Geometry: final body of the model. Coordinates: model frame, mm. Face numbers are marked on the shaded views. A direction names the side the tool comes from. Coordinates: 2 decimals unless noted, no trailing zeros. Order: outer loops, then holes, each group sorted by start corner. A loop starts at its lowest first (then second) coordinate and runs counter-clockwise, first axis right, second up. Notation, with made-up numbers: (58, -32.5) - (71, -32.5) arc R36 cw to (71, 6.5) - close; hole circle Ø11 at (48.25, 27.5). An arc over 180 degrees is marked (long way). Use one line per item in the form item = value. Start each with the question number.
```python
from build123d import *

# Parameters (mm, degrees)
SKETCH1_W                 = 50.8
SKETCH1_H                 = 50.8
SKETCH1_W_2               = 38.1
SKETCH1_H_2               = 38.1
BOSS_EXTRUDE1_DEPTH       = 178
SKETCH2_W                 = 44.8
SKETCH2_H                 = 44.8
SKETCH2_W_2               = 38.1
SKETCH2_H_2               = 38.1
CUT_EXTRUDE1_DEPTH        = 20
SKETCH3_W                 = 46.8
SKETCH3_H                 = 123.47500012
CUT_EXTRUDE2_DEPTH        = 47.625
CUT_EXTRUDE5_DEPTH        = 1
SKETCH7_W                 = 46.8
SKETCH7_H                 = 3.675
CUT_EXTRUDE6_DEPTH        = 1
FILLET1_R                 = 1.5875
CUT_EXTRUDE7_REACH        = 193.951
F_0_80_TAPPED_HOLE1_D     = 1.19126
F_0_80_TAPPED_HOLE1_DEPTH = 2.9997
F_0_80_TAPPED_HOLE1_TIP   = 0.357890611
SKETCH19_W                = 50.8
SKETCH19_H                = 1.5875
CUT_EXTRUDE12_DEPTH       = 4
CIRPATTERN1_COUNT         = 4
CUT_EXTRUDE13_DEPTH       = 191.931610793
LPATTERN1_COUNT           = 2
LPATTERN1_PITCH           = 8.41
LPATTERN1_COPY_1_SKETCH_W = 50.8
LPATTERN1_COPY_1_SKETCH_H = 1.5875
LPATTERN1_COPY_1_DEPTH    = 4
LPATTERN1_COPY_2_SKETCH_W = 50.8
LPATTERN1_COPY_2_SKETCH_H = 1.5875
LPATTERN1_COPY_2_DEPTH    = 4
LPATTERN1_COPY_3_SKETCH_W = 50.8
LPATTERN1_COPY_3_SKETCH_H = 1.5875
LPATTERN1_COPY_3_DEPTH    = 4


with BuildPart() as part:
    # Sketch1 → Boss-Extrude1 (new body)
    with BuildSketch(Plane(origin=(0, 0, 0), x_dir=(1, 0, 0), z_dir=(0, 1, 0))):
        with Locations((25.4, 25.4)):
            Rectangle(SKETCH1_W, SKETCH1_H)
        with Locations((25.4, 25.4)):
            Rectangle(SKETCH1_W_2, SKETCH1_H_2, mode=Mode.SUBTRACT)
    extrude(amount=BOSS_EXTRUDE1_DEPTH)

    # Sketch2 → Cut-Extrude1 (cut)
    with BuildSketch(Plane.XZ):
        with Locations((25.4, -25.4)):
            Rectangle(SKETCH2_W, SKETCH2_H)
        with Locations((25.4, -25.4)):
            Rectangle(SKETCH2_W_2, SKETCH2_H_2, mode=Mode.SUBTRACT)
    extrude(amount=-CUT_EXTRUDE1_DEPTH, mode=Mode.SUBTRACT)

    # Sketch3 → Cut-Extrude2 (cut)
    with BuildSketch(Plane.XY):
        with Locations((25.4, 109.41249994)):
            Rectangle(SKETCH3_W, SKETCH3_H)
    extrude(amount=-CUT_EXTRUDE2_DEPTH, mode=Mode.SUBTRACT)

    # Sketch6 → Cut-Extrude5 (cut)
    with BuildSketch(Plane.ZY):
        with BuildLine():
            Line((-32.4, 171.5), (-18.4, 171.5))
            ThreePointArc((-18.4, 171.5), (-17.4, 170.5), (-18.4, 169.5))
            Line((-18.4, 169.5), (-32.4, 169.5))
            ThreePointArc((-32.4, 169.5), (-33.4, 170.5), (-32.4, 171.5))
        make_face()
        with BuildLine():
            Line((-32.4, 168), (-18.4, 168))
            ThreePointArc((-18.4, 168), (-17.4, 167), (-18.4, 166))
            Line((-18.4, 166), (-32.4, 166))
            ThreePointArc((-32.4, 166), (-33.4, 167), (-32.4, 168))
        make_face()
        with BuildLine():
            Line((-32.4, 164.5), (-18.4, 164.5))
            ThreePointArc((-18.4, 164.5), (-17.4, 163.5), (-18.4, 162.5))
            Line((-18.4, 162.5), (-32.4, 162.5))
            ThreePointArc((-32.4, 162.5), (-33.4, 163.5), (-32.4, 164.5))
        make_face()
    cut_extrude5 = extrude(amount=-CUT_EXTRUDE5_DEPTH, mode=Mode.SUBTRACT)

    # Mirror2: Cut-Extrude5 across plane
    add(cut_extrude5.mirror(Plane.ZY.offset(-25.4)), mode=Mode.SUBTRACT)

    # Sketch7 → Cut-Extrude6 (cut)
    with BuildSketch(Plane.XY):
        with Locations((25.4, 172.9875)):
            Rectangle(SKETCH7_W, SKETCH7_H)
        with Locations((25.4, 45.83749988)):
            Rectangle(SKETCH7_W, SKETCH7_H)
    extrude(amount=-CUT_EXTRUDE6_DEPTH, mode=Mode.SUBTRACT)

    # Fillet1
    fillet1_edges = [part.edges().sort_by_distance(p)[0] for p in [
        (2, 174.825, -0.5),
        (48.8, 174.825, -0.5),
        (2, 43.99999988, -0.5),
        (48.8, 43.99999988, -0.5),
        (47.8, 10, -3),
        (47.8, 10, -47.8),
        (3, 10, -47.8),
        (3, 10, -3),
        (2, 47.67499988, -24.3125),
        (2, 171.15, -24.3125),
        (48.8, 171.15, -24.3125),
        (48.8, 47.67499988, -24.3125),
    ]]
    fillet(fillet1_edges, radius=FILLET1_R)

    # Sketch8 → Cut-Extrude7 (cut, up to next)
    with BuildSketch(Plane(origin=(0, 178, 0), x_dir=(1, 0, 0), z_dir=(0, 1, 0)), mode=Mode.PRIVATE) as cut_extrude7_sk1:
        with BuildLine():
            Line((6.9375, 45.45), (43.8625, 45.45))
            ThreePointArc((43.8625, 45.45), (44.985032015, 44.985032015), (45.45, 43.8625))
            Line((45.45, 43.8625), (45.45, 6.9375))
            ThreePointArc((45.45, 6.9375), (44.985032015, 5.814967985), (43.8625, 5.35))
            Line((43.8625, 5.35), (6.9375, 5.35))
            ThreePointArc((6.9375, 5.35), (5.814967985, 5.814967985), (5.35, 6.9375))
            Line((5.35, 6.9375), (5.35, 43.8625))
            ThreePointArc((5.35, 43.8625), (5.814967985, 44.985032015), (6.9375, 45.45))
        make_face()
    cut_extrude7_tool1 = extrude(cut_extrude7_sk1.sketch, amount=-CUT_EXTRUDE7_REACH, mode=Mode.PRIVATE) & part.part
    add(cut_extrude7_tool1.solids().sort_by_distance((25.4, 178, -25.4))[0], mode=Mode.SUBTRACT)

    # 0-80 Tapped Hole1
    with Locations(Plane.XY.offset(-1)):
        with Locations((4.25425, 172.571000052), (46.51375, 172.571000052), (4.25425, 46.285999828), (46.51375, 46.285999828)):
            Hole(F_0_80_TAPPED_HOLE1_D / 2, depth=F_0_80_TAPPED_HOLE1_DEPTH)
            with Locations((0, 0, -(F_0_80_TAPPED_HOLE1_DEPTH + F_0_80_TAPPED_HOLE1_TIP / 2))):  # 118° drill point
                Cone(0, F_0_80_TAPPED_HOLE1_D / 2, F_0_80_TAPPED_HOLE1_TIP, mode=Mode.SUBTRACT)

    # Sketch19 → Cut-Extrude12 (cut)
    with BuildSketch(Plane.XY):
        with Locations((25.4, 24.79375)):
            Rectangle(SKETCH19_W, SKETCH19_H)
    cut_extrude12 = extrude(amount=-CUT_EXTRUDE12_DEPTH, mode=Mode.SUBTRACT)

    # CirPattern1: Cut-Extrude12 ×4 about axis
    cirpattern1_axis = Axis((25.4, 0, -25.4), (0, 1, 0))
    for i in range(1, CIRPATTERN1_COUNT):
        add(cut_extrude12.rotate(cirpattern1_axis, i * 360 / CIRPATTERN1_COUNT), mode=Mode.SUBTRACT)

    # Sketch20 → Cut-Extrude13 (cut, through all)
    with BuildSketch(Plane(origin=(46.8, 0, -50.8), x_dir=(0, 0, 1), z_dir=(-1, 0, 0))):
        with BuildLine():
            Line((11.19375, 25.5875), (39.60625, 25.5875))
            ThreePointArc((39.60625, 25.5875), (40.4, 24.79375), (39.60625, 24))
            Line((39.60625, 24), (11.19375, 24))
            ThreePointArc((11.19375, 24), (10.4, 24.79375), (11.19375, 25.5875))
        make_face()
    cut_extrude13 = extrude(amount=CUT_EXTRUDE13_DEPTH, mode=Mode.SUBTRACT)

    # LPattern1: Cut-Extrude12, Cut-Extrude13 ×2
    with Locations(*[(0, i * LPATTERN1_PITCH, 0) for i in range(1, LPATTERN1_COUNT)]):
        add(cut_extrude12, mode=Mode.SUBTRACT)
        add(cut_extrude13, mode=Mode.SUBTRACT)

    # LPattern1 copy 1 sketch → LPattern1 copy 1 (cut)
    with BuildSketch(Plane(origin=(50.8, 8.41, 0), x_dir=(0, 0, -1), z_dir=(1, 0, 0))):
        with Locations((25.4, 24.79375)):
            Rectangle(LPATTERN1_COPY_1_SKETCH_W, LPATTERN1_COPY_1_SKETCH_H)
    extrude(amount=-LPATTERN1_COPY_1_DEPTH, mode=Mode.SUBTRACT)

    # LPattern1 copy 2 sketch → LPattern1 copy 2 (cut)
    with BuildSketch(Plane(origin=(50.8, 8.41, -50.8), x_dir=(-1, 0, 0), z_dir=(0, 0, -1))):
        with Locations((25.4, 24.79375)):
            Rectangle(LPATTERN1_COPY_2_SKETCH_W, LPATTERN1_COPY_2_SKETCH_H)
    extrude(amount=-LPATTERN1_COPY_2_DEPTH, mode=Mode.SUBTRACT)

    # LPattern1 copy 3 sketch → LPattern1 copy 3 (cut)
    with BuildSketch(Plane(origin=(0, 8.41, -50.8), x_dir=(0, 0, 1), z_dir=(-1, 0, 0))):
        with Locations((25.4, 24.79375)):
            Rectangle(LPATTERN1_COPY_3_SKETCH_W, LPATTERN1_COPY_3_SKETCH_H)
    extrude(amount=-LPATTERN1_COPY_3_DEPTH, mode=Mode.SUBTRACT)


solid = part.part
```
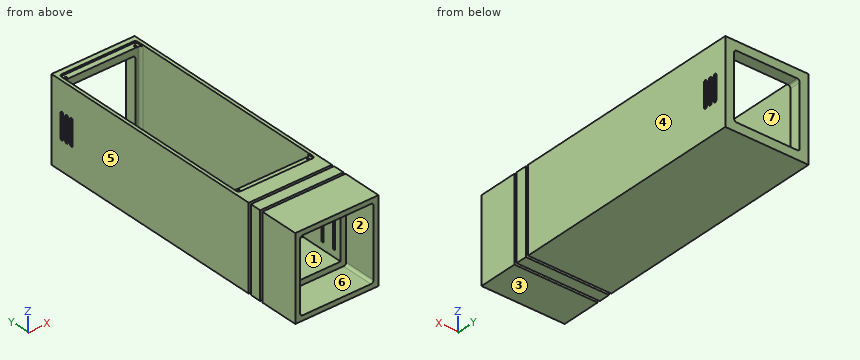
(1) Draft query along X for the marked faces 1, 2, 3 and 4. Return one class per face: released by +X, released by -X, zero draft, split by the parting line, or undercut.
(2) Cut plane B-B on z = -14. Count the separate pieces of the cut face and the enclosed holes in it, plus the area to 3 significant figures.
(3) Contact query for flat-ended pins moving along their axis: pin 1 Ø10 at (x, z) = (35, -11) entering from +Y (3 decimals); pin 2 Ø1 at (x, y) = (35.5, 68) entering from +Z (3 decimals); pin 3 Ø0.8 at (y, z) = (33.5, -8.5) entering from -X; pin 4 Ø15 at (x, z) = (35.5, -26) entering from -Y. Output: stop coordinate, or through.
(4) Cut plane A-A on y = 108.5. Return the cut outline in (x, z) (3 decimals), plus the area to 3 significant figures.
(5) Set-up query: the marked faces 5, 6 and 7. Return all of +Z, -Z, +X, -X, +Y, -Y with unobstructed straight access to the full face (end or side cutting, diameter ignored); none if empty.
(6) Material intervals for L1, parallel to X at y = 136, z = -6; L2, parallel to Z at x = 19.5, y = 10; L3, parallel to X at y = 37, z = -9, sorted ascending. Write a range as from..to.
Check sheet entries:
q1.face_1 = undercut
q1.face_2 = undercut
q1.face_3 = zero draft
q1.face_4 = released by +X
q2.separate_pieces = 6
q2.enclosed_holes = 0
q2.area = 1,000 mm^2
q3.pin_1 = 47.675
q3.pin_2 = -47.625
q3.pin_3 = 4
q3.pin_4 = through
q4.outline = (0, -50.8) - (50.8, -50.8) - (50.8, 0) - (48.8, 0) - (48.8, -47.625) - (2, -47.625) - (2, 0) - (0, 0) - close
q4.area = 352 mm^2
q5.face_5 = +Z, -Z, -X, +Y, -Y
q5.face_6 = -Y
q5.face_7 = +Z
q6.L1 = 0..2, 48.8..50.8
q6.L2 = -50.8..-47.8, -3..0
q6.L3 = 0..6.35, 44.45..50.8
